```python
from build123d import *

# Parameters (mm, degrees)
EXTRUDE_1_DEPTH = 2


with BuildPart() as part:
    # 草圖1 → 旋轉1 (revolve)
    with BuildSketch(Plane.XY):
        Polygon((0, 0), (55, 0), (55, -16), (58.5, -16), (58.5, -23), (45, -23), (45, -37), (10, -37), (10, -57), (5, -57), (5, -39), (0, -39), align=None)
    revolve(axis=Axis((0, 84.440513305, 0), (0, -1, 0)))

    # 草圖3 → 填料-伸長1 (add)
    with BuildSketch(Plane(origin=(0, 0, 0), x_dir=(1, 0, 0), z_dir=(0, 1, 0))):
        with BuildLine():
            Line((-20, 51.23475383), (-20, -51.23475383))
            ThreePointArc((-20, -51.23475383), (0, -55), (20, -51.23475383))
            Line((20, -51.23475383), (20, 51.23475383))
            ThreePointArc((20, 51.23475383), (0, 55), (-20, 51.23475383))
        make_face()
    extrude(amount=EXTRUDE_1_DEPTH)


solid = part.part
```
Part model, mm, in its own coordinate system. A direction names the side the tool comes from. Round coordinates to 2 decimals unless told otherwise and drop trailing zeros. Write each loop counter-clockwise with the first axis right and the second up, starting at its lowest first coordinate (ties: lowest second). Pieces come first, ordered by that corner, then holes.
Item 1: Cut at C-C, the plane y = -43. Give the cut face in (x, z), plus the area to 3 significant figures.
Results:
outline: circle Ø20 at (0, 0); hole circle Ø10 at (0, 0)
area: 236 mm2
Item 2: Cut at D-D, the plane y = -13. Give the cut face in (x, z).
Results:
outline: circle Ø110 at (0, 0)
Item 3: Cut at B-B, the plane x = 0. Give the cut face in (y, z).
Results:
outline: (-57, -10) - (-37, -10) - (-37, -45) - (-23, -45) - (-23, -58.5) - (-16, -58.5) - (-16, -55) - (2, -55) - (2, 55) - (-16, 55) - (-16, 58.5) - (-23, 58.5) - (-23, 45) - (-37, 45) - (-37, 10) - (-57, 10) - (-57, 5) - (-39, 5) - (-39, -5) - (-57, -5) - close
Item 4: Drop flat-ended pins along their axis: pin 1 Ø8 at (x, z) = (-8, -29.5) entering from -Y; pin 2 Ø10 at (x, y) = (16.5, -25) entering from +Z; pin 3 Ø1 at (y, z) = (-22.5, -14.5) entering from -X; pin 4 Ø8 at (x, z) = (1, -2) entering from -Y. Give the stop position or say it passes through.
Results:
pin 1: stops at y = -37
pin 2: stops at z = 57.27
pin 3: stops at x = -56.8
pin 4: stops at y = -57
Item 5: Two-plate mould, pull along X, no slides. Class faces 1 (the flat face through (34, 0, 1)), 2 (the cylindrical face through (20.765, -30.098, -39.923)), 3 (the flat face through (0, -39, 0)): +X half, -X half, draft (parallel to the pull), parting line (faces both ways), or undercut.
Results:
face 1: draft
face 2: parting line
face 3: undercut
Item 6: Which spindle directions (+Z, -Z, +X, -X, +Y, -Y) get a long thin tool onto all of the face, cutting with end or side? Do faces 4 (the flat face through (-39, -16, 39)), 5 (the flat face through (30, -23, -34)), 6 (the flat face through (-33, 0, 1)), 7 (the flat face through (0, 2, -1)), 8 (the cylindrical face through (-12.68, -19.55, -57.11)). Say none if no direction does.
Results:
face 4: +Y
face 5: -Y
face 6: +Z, -Z, -X, +Y
face 7: +Z, -Z, +X, -X, +Y
face 8: +Y, -Y
Item 7: Probe L1, parallel to Z at x = 0, y = -47; L2, parallel to Y at x = -41.5, z = -6; L3, parallel to Y at x = 5.5, z = 45. List the from-to ranges inside material, lowest first.
Results:
L1: z = -10 to -5, 5 to 10
L2: y = -37 to 0
L3: y = -23 to 2
Item 8: Cut at A-A, the plane z = 0. Give the cut face in (x, y), plus the area to 3 significant figures.
Results:
outline: (-58.5, -23) - (-45, -23) - (-45, -37) - (-10, -37) - (-10, -57) - (-5, -57) - (-5, -39) - (5, -39) - (5, -57) - (10, -57) - (10, -37) - (45, -37) - (45, -23) - (58.5, -23) - (58.5, -16) - (55, -16) - (55, 0) - (20, 0) - (20, 2) - (-20, 2) - (-20, 0) - (-55, 0) - (-55, -16) - (-58.5, -16) - close
area: 4,140 mm2
